The model under review builds one solid part; all positions refer to its coordinate system, in mm. A direction names the side the tool comes from. Coordinates: 2 decimals unless noted, no trailing zeros. Loops run counter-clockwise (first coordinate to the right, second up) from the corner with the lowest first, then second, coordinate; pieces in that order, holes last. Notation, with made-up numbers: M 67.25,16.5 L 86.25,16.5 A23 ccw 86.25,38.5 Z; hole C 59,-25.75 d1. An arc over 180 degrees is marked long. Use CSV: the item, a comma, the result in double quotes. Start each with the question number.
1. Draft analysis for pull direction Y (two halves, no side actions). For faces 1 (the flat face through (-10, 11, 0)), 2 (the cylindrical face through (-1.5, 0.07, 10.58)), 3 (the flat face through (-15, -7, 5)), state which applies: +Y half, -Y half, draft (parallel to the pull), parting line (faces both ways), or undercut.
2. Add section A-A, the plane y = -6.75. Write out the cut boundary in (x, z).
3. Add section B-B, the plane z = -4.75. Write out the cut boundary in (x, y).
4. For L1, parallel to X at y = -6.25, z = 7.5; L2, parallel to X at y = 8, z = 1.5; L3, parallel to Y at x = 0, z = 10.4, list the stretches that pass through material, from the lowest coordinate up.
5. Add section D-D, the plane x = 7.25. Write out the cut boundary in (y, z), then the cut area to 3 significant figures.
6. Add section C-C, the plane x = 0. Write out the cut boundary in (y, z).
7. Tool access review of faces 4 (the flat face through (-14, -3, 5)), 5 (the flat face through (-13, -8, 0)), 6 (the flat face through (0, -3, 9.4)), 7 (the cylindrical face through (-12.49, -7.75, 5.58)): name each direction out of +Z, -Z, +X, -X, +Y, -Y from which nothing blocks a thin tool from reaching the whole face with its end or side.
8. Clearance check with flat-ended pins moving along their axes: P1, Ø5.5, axis at y = 2.5, z = -1.5, coming from the -X side; P2, Ø1.4, axis at x = -14, z = 6, coming from the +Y side; P3, Ø2.5, axis at x = 0, y = 0, coming from the +Z side. State where each tip first meets the part, or that it passes through.
from build123d import *

# Parameters (mm, degrees)
F0_W     = 22
F0_H     = 22
F0_W_2   = 18.8
F0_H_2   = 18.8
F1_DEPTH = 11
F2_R     = 1.5
F3_DEPTH = 25
F4_SIZE  = 0.75
F6_DEPTH = 11
F7_R     = 0.87499
F8_SIZE  = 1


# Not quite as in the source:
# - a fillet or chamfer is up to 0.001 mm smaller than in the source, because OpenCascade refuses the exact size


with BuildPart() as f1:
    # F0 (on Front) → F1 (new body, symmetric)
    with BuildSketch(Plane.XZ):
        Rectangle(F0_W, F0_H)
        Rectangle(F0_W_2, F0_H_2, mode=Mode.SUBTRACT)
    extrude(amount=F1_DEPTH, both=True)

    # F2 (on face) → F3 (cut)
    with BuildSketch(Plane.XY.offset(11)):
        Circle(F2_R)
    extrude(amount=-F3_DEPTH, mode=Mode.SUBTRACT)

    # F4
    f4_edges = [f1.edges().sort_by_distance(p)[0] for p in [
        (-1.5, 0, -9.4),
        (-1.5, 0, 9.4),
    ]]
    chamfer(f4_edges, length=F4_SIZE)

    # F5 (on Top) → F6 (join, through all)
    with BuildSketch(Plane.XY):
        Polygon((-12.75, -3), (-15, -3), (-15, -11), (-11, -11), (-11, -8), (-12.75, -8), align=None)
    extrude(amount=F6_DEPTH)

    # F7 (radius 0.875 in the source; OpenCascade refuses exactly that, so slightly less here)
    f7_edges = [f1.edges().sort_by_distance(p)[0] for p in [
        (-12.75, -8, 5.5),
        (-11, -8, 5.5),
    ]]
    fillet(f7_edges, radius=F7_R)

    # F8
    f8_edges = [f1.edges().sort_by_distance(p)[0] for p in [
        (-12.75, -3, 5.5),
    ]]
    chamfer(f8_edges, length=F8_SIZE)


solid = f1.part
Computed:
1,face 1,"+Y half"
1,face 2,"undercut"
1,face 3,"draft"
2,outline,"M -15,0 L -12.75,0 L -12.75,11 L -15,11 Z; M -11,-11 L 11,-11 L 11,11 L -11,11 Z; hole M -9.4,-9.4 L 9.4,-9.4 L 9.4,9.4 L -9.4,9.4 Z"
3,outline,"M -11,-11 L -9.4,-11 L -9.4,11 L -11,11 Z; M 9.4,-11 L 11,-11 L 11,11 L 9.4,11 Z"
4,L1,"x = -15 to -12.75, -11 to -9.4, 9.4 to 11"
4,L2,"x = -11 to -9.4, 9.4 to 11"
4,L3,"y = -11 to -1.5, 1.5 to 11"
5,outline,"M -11,-11 L 11,-11 L 11,-9.4 L -11,-9.4 Z; M -11,9.4 L 11,9.4 L 11,11 L -11,11 Z"
5,area,"70.4 mm^2"
6,outline,"M -11,-11 L -1.5,-11 L -1.5,-10.15 L -2.25,-9.4 L -11,-9.4 Z; M -11,9.4 L -2.25,9.4 L -1.5,10.15 L -1.5,11 L -11,11 Z; M 1.5,-11 L 11,-11 L 11,-9.4 L 2.25,-9.4 L 1.5,-10.15 Z; M 1.5,10.15 L 2.25,9.4 L 11,9.4 L 11,11 L 1.5,11 Z"
7,face 4,"+Z, -Z, -X, +Y"
7,face 5,"-Z, -X, +Y, -Y"
7,face 6,"+Y, -Y"
7,face 7,"+Z, -Z, +Y"
8,P1,"stops at x = -11"
8,P2,"stops at y = -3"
8,P3,"passes through"
